Build history of the part. All positions in model axes, mm. Face numbers are marked on the shaded views. A direction names the side the tool comes from. Round coordinates to 2 decimals unless told otherwise and drop trailing zeros. Loops run counter-clockwise (first coordinate to the right, second up) from the corner with the lowest first, then second, coordinate; pieces in that order, holes last.
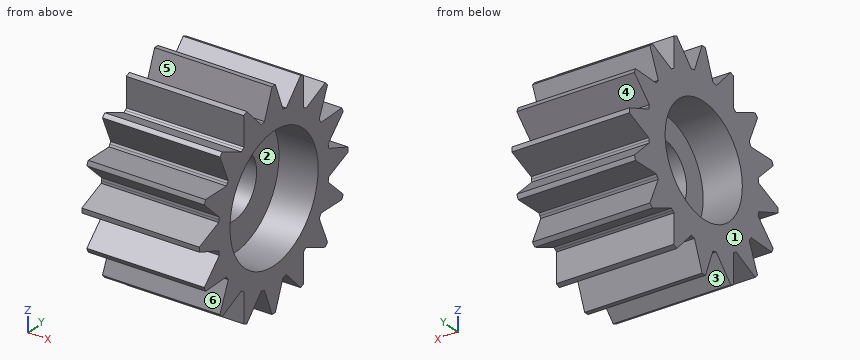
from build123d import *

# Parameters (mm, degrees)
F0_R            = 13.5
F1_DEPTH        = 15
F2_R            = 7
F3_DEPTH        = 5
F5_DEPTH        = 15.001
F5_COPIES_COUNT = 16
F6_R            = 8
F7_DEPTH        = 5
F8_R            = 4
F9_DEPTH        = 10.001


# Not quite as in the source:
# - a pattern or mirror of a feature is missing from the dataset's text; its kind, count and spacing are read off the source's solid


with BuildPart() as f1:
    # F0 (on Right) → F1 (new body)
    with BuildSketch(Plane.YZ):
        Circle(F0_R)
    extrude(amount=-F1_DEPTH)

    # F2 (on face) → F3 (cut)
    with BuildSketch(Plane(origin=(-15, 0, 0), x_dir=(0, -1, 0), z_dir=(-1, 0, 0))):
        Circle(F2_R)
    extrude(amount=-F3_DEPTH, mode=Mode.SUBTRACT)

    # F4 (on face) → F5 (cut, through all)
    with BuildSketch(Plane(origin=(-15, 0, 0), x_dir=(0, -1, 0), z_dir=(-1, 0, 0))):
        with BuildLine():
            Line((2.2686257354, 9.8675712449), (4.8878039751, 12.5840920332))
            ThreePointArc((4.8878039751, 12.5840920332), (2.6337193472, 13.2406012854), (0.2999814809, 13.4966666667))
            Line((0.2999814809, 13.4966666667), (1.6802191492, 9.9846125919))
            Line((1.6802191492, 9.9846125919), (1.9752895104, 9.9304509641))
            Line((1.9752895104, 9.9304509641), (2.2686257354, 9.8675712449))
        make_face()
    f5 = extrude(amount=-F5_DEPTH, mode=Mode.SUBTRACT)

    # F5_copies: F5 ×16 about axis
    f5_copies_axis = Axis((0, 0, 0), (1, 0, 0))
    for i in range(1, F5_COPIES_COUNT):
        add(f5.rotate(f5_copies_axis, i * 360 / F5_COPIES_COUNT), mode=Mode.SUBTRACT)

    # F6 (on face) → F7 (cut)
    with BuildSketch(Plane.YZ):
        with Locations((0.0570340926, 0.13036374)):
            Circle(F6_R)
    extrude(amount=-F7_DEPTH, mode=Mode.SUBTRACT)

    # F8 (on face) → F9 (cut, through all)
    with BuildSketch(Plane.YZ.offset(-5)):
        Circle(F8_R)
    extrude(amount=-F9_DEPTH, mode=Mode.SUBTRACT)


solid = f1.part
(1) Probe line 1 (Z direction, x = -7.05, y = 0); line 2 (Z direction, x = -12.35, y = 0); line 3 (Z direction, x = -10.5, y = -9.5). List the from-to ranges inside material, lowest first.
Responses:
line 1: z = -13.5 to -4, 4 to 13.5
line 2: z = -13.5 to -7, 7 to 13.5
line 3: z = -9.59 to -8.74, -5.39 to 5.39, 8.74 to 9.59
(2) Which spindle directions (+Z, -Z, +X, -X, +Y, -Y) get a long thin tool onto all of the face, cutting with end or side? Do the marked faces 4, 5 and 6. Say none if no direction does.
Responses:
face 4: +X, -X, +Y
face 5: +Z, +X, -X
face 6: +X, -X, -Y
(3) Slice it at B-B on y = 11. List the corners of the cut face in (x, z), plus the area to 3 significant figures.
Responses:
outline: (-15, -5.42) - (0, -5.42) - (0, -3.36) - (-15, -3.36) - close; (-15, -1.28) - (0, -1.28) - (0, 1.28) - (-15, 1.28) - close; (-15, 3.36) - (0, 3.36) - (0, 5.42) - (-15, 5.42) - close
area: 100 mm2
(4) Pin check, flat tips, straight feed: P1, Ø6, axis at x = -7.5, z = -4, coming from the +Y side; P2, Ø1.5, axis at x = -7.5, y = 9.5, coming from the +Z side; P3, Ø4, axis at y = -3.5, z = -1.5, coming from the -X side; P4, Ø6.5, axis at y = 0, z = 0, coming from the +X side. Stop position of each tip, or through.
Responses:
P1: stops at y = 12.58
P2: stops at z = 9.76
P3: stops at x = -10
P4: passes through
(5) Pull direction Z, two halves, no side cores. Call the marked faces 1, 2 and 3: +Z half, -Z half, draft (parallel to the pull), parting line (faces both ways), or undercut.
Responses:
face 1: draft
face 2: undercut
face 3: -Z half
(6) Slice it at A-A on y = -3.5. List the corners of the cut face in (x, z), plus the area to 3 significant figures.
Responses:
outline: (-15, -11.14) - (0, -11.14) - (0, -7.04) - (-5, -7.04) - (-5, -1.94) - (-10, -1.94) - (-10, -6.06) - (-15, -6.06) - close; (-15, 6.06) - (-10, 6.06) - (-10, 1.94) - (-5, 1.94) - (-5, 7.3) - (0, 7.3) - (0, 11.14) - (-15, 11.14) - close
area: 183 mm2
